Can you work these out from the model? Positions are in its coordinate system, mm. A direction names the side the tool comes from. Coordinates: 2 decimals unless noted, no trailing zeros. Order: outer loops, then holes, each group sorted by start corner. A loop starts at its lowest first (then second) coordinate and runs counter-clockwise, first axis right, second up. Notation, with made-up numbers: (35.25, 35.5) -> (71.25, 35.5) arc R22 cw to (71.25, 46.5) -> close; hole circle Ø2 at (41, 27.25). An arc over 180 degrees is marked (long way). Answer as a JSON object with one key per item and string values. Group by question number.
(1) I want a section at A-A, the plane y = 19. List the corners of the cut face in (x, z) for me.
(2) I need wall thicknesses on line 1 (X direction, y = 6, z = -98); line 2 (Z direction, x = 31, y = 9); line 3 (X direction, y = 10, z = -106). Which ranges of each line are inside material? Lowest first, please.
(3) I want a section at C-C, the plane x = -12. List the corners of the cut face in (y, z) for me, plus the area to 3 significant figures.
(4) I want a section at B-B, the plane z = 91.5. List the corners of the cut face in (x, y) for me, plus the area to 3 significant figures.
(5) Which directions (+Z, -Z, +X, -X, +Y, -Y) give clear straight access to the entire face, cutting with the end or side of a thin tool? Please do faces 4 (the flat face through (-108, 7, 1)), 5 (the flat face through (-1, 7, -116)), 6 (the flat face through (-110, 1, 1)).
(6) If we mould it in two halves opening along X, with no side actions, what happens to faces 1 (the flat face through (-102.6, 17.2, 112.4)), 2 (the flat face through (110, 1, 1)), 3 (the flat face through (95, 14, -109))? For each: pulls with the +X half, pulls with the -X half, needs draft (parallel to the pull), parting line crosses it, or undercut.
(7) For pin 1 (16.5 mm diameter, centred on x = -105.5, y = 21.5, fed in from -Z) (3 decimals); pin 2 (0.6 mm diameter, centred on x = -108.5, z = 14.5, fed in from +Y); pin 3 (1.5 mm diameter, centred on y = 12.5, z = 38.5, fed in from -X), each with a flat end and sliding along its axis, tell me the tip position at first contact or that it passes through.
from build123d import *

# Parameters (mm, degrees)
SKETCH2_W           = 220
SKETCH2_H           = 240
BOSS_EXTRUDE1_DEPTH = 2
SKETCH4_W           = 190
SKETCH4_H           = 2
SKETCH4_W_2         = 2
SKETCH4_H_2         = 210
BOSS_EXTRUDE3_DEPTH = 10
BOSS_EXTRUDE4_DEPTH = 15
BOSS_EXTRUDE5_DEPTH = 15


with BuildPart() as part:
    # Sketch2 → Boss-Extrude1 (new body)
    with BuildSketch(Plane(origin=(0, 0, 0), x_dir=(1, 0, 0), z_dir=(0, 1, 0))):
        Rectangle(SKETCH2_W, SKETCH2_H)
    extrude(amount=BOSS_EXTRUDE1_DEPTH)

    # Sketch4 → Boss-Extrude3 (add)
    with BuildSketch(Plane(origin=(0, 2, 0), x_dir=(1, 0, 0), z_dir=(0, 1, 0))):
        with Locations((0, 117)):
            Rectangle(SKETCH4_W, SKETCH4_H)
        with Locations((-107, 0)):
            Rectangle(SKETCH4_W_2, SKETCH4_H_2)
        with Locations((0, -117)):
            Rectangle(SKETCH4_W, SKETCH4_H)
        with Locations((107, 0)):
            Rectangle(SKETCH4_W_2, SKETCH4_H_2)
    extrude(amount=BOSS_EXTRUDE3_DEPTH)

    # Sketch5 → Boss-Extrude4 (add)
    with BuildSketch(Plane(origin=(110, 0, 0), x_dir=(0, 0, -1), z_dir=(1, 0, 0))):
        Polygon((-120, 2), (-105, 2), (-105, 32), align=None)
        Polygon((120, 2), (105, 2), (105, 32), align=None)
    extrude(amount=-BOSS_EXTRUDE4_DEPTH)

    # Sketch6 → Boss-Extrude5 (add)
    with BuildSketch(Plane.ZY.offset(110)):
        Polygon((120, 2), (105, 2), (105, 32), align=None)
        Polygon((-105, 32), (-105, 2), (-120, 2), align=None)
    extrude(amount=-BOSS_EXTRUDE5_DEPTH)


solid = part.part
Computed values:
{
 "1": {"outline": "(-110, -111.5) -> (-95, -111.5) -> (-95, -105) -> (-110, -105) -> close; (-110, 105) -> (-95, 105) -> (-95, 111.5) -> (-110, 111.5) -> close; (95, -111.5) -> (110, -111.5) -> (110, -105) -> (95, -105) -> close; (95, 105) -> (110, 105) -> (110, 111.5) -> (95, 111.5) -> close"},
 "2": {"line 1": "x = -108 to -106, 106 to 108", "line 2": "z = -118 to -116, 116 to 118", "line 3": "x = -110 to -95, 95 to 110"},
 "3": {"outline": "(0, -120) -> (2, -120) -> (2, -118) -> (12, -118) -> (12, -116) -> (2, -116) -> (2, 116) -> (12, 116) -> (12, 118) -> (2, 118) -> (2, 120) -> (0, 120) -> close", "area": "520 mm2"},
 "4": {"outline": "(-110, 0) -> (110, 0) -> (110, 2) -> (108, 2) -> (108, 12) -> (106, 12) -> (106, 2) -> (-106, 2) -> (-106, 12) -> (-108, 12) -> (-108, 2) -> (-110, 2) -> close", "area": "480 mm2"},
 "5": {"face 4": "-X, +Y", "face 5": "+Y", "face 6": "+Z, -Z, -X, +Y, -Y"},
 "6": {"face 1": "needs draft", "face 2": "pulls with the +X half", "face 3": "undercut"},
 "7": {"pin 1": "stops at z = -114.375", "pin 2": "stops at y = 2", "pin 3": "stops at x = -108"}
}
